from build123d import *

# Parameters (mm, degrees)
F1_DEPTH = 15
F3_DEPTH = 10


with BuildPart() as f1:
    # F0 (on Front) → F1 (new body)
    with BuildSketch(Plane.XZ):
        Polygon((-28.551763, 0), (-7.551763, 0), (-7.551763, 2), (-8.551763, 2), (-8.551763, 3), (-27.551763, 3), (-27.551763, 2), (-28.551763, 2), align=None)
    extrude(amount=F1_DEPTH)

    # F2 (on face) → F3 (cut)
    with BuildSketch(Plane(origin=(0, 0, 0), x_dir=(-1, 0, 0), z_dir=(0, 1, 0))):
        Polygon((8.051763, 1.5), (8.051763, 0.5), (9.301763, 0.5), (9.301763, 1), (9.801763, 1), (9.801763, 0.5), (10.301763, 0.5), (10.301763, 1), (10.801763, 1), (10.801763, 0.5), (11.301763, 0.5), (11.301763, 1), (11.801763, 1), (11.801763, 0.5), (12.301763, 0.5), (12.301763, 1), (12.801763, 1), (12.801763, 0.5), (13.301763, 0.5), (13.301763, 1), (13.801763, 1), (13.801763, 0.5), (14.301763, 0.5), (14.301763, 1), (14.801763, 1), (14.801763, 0.5), (15.301763, 0.5), (15.301763, 1), (15.801763, 1), (15.801763, 0.5), (16.301763, 0.5), (16.301763, 1), (16.801763, 1), (16.801763, 0.5), (17.301763, 0.5), (17.301763, 1), (17.801763, 1), (17.801763, 0.5), (18.301763, 0.5), (18.301763, 1), (18.801763, 1), (18.801763, 0.5), (19.301763, 0.5), (19.301763, 1), (19.801763, 1), (19.801763, 0.5), (20.301763, 0.5), (20.301763, 1), (20.801763, 1), (20.801763, 0.5), (21.301763, 0.5), (21.301763, 1), (21.801763, 1), (21.801763, 0.5), (22.301763, 0.5), (22.301763, 1), (22.801763, 1), (22.801763, 0.5), (23.301763, 0.5), (23.301763, 1), (23.801763, 1), (23.801763, 0.5), (24.301763, 0.5), (24.301763, 1), (24.801763, 1), (24.801763, 0.5), (25.301763, 0.5), (25.301763, 1), (25.801763, 1), (25.801763, 0.5), (26.301763, 0.5), (26.301763, 1), (26.831981, 1), (26.831981, 0.5), (28.081981, 0.5), (28.081981, 1.5), (27.081981, 1.5), (27.081981, 2.5), (26.301763, 2.5), (26.301763, 2), (25.801763, 2), (25.801763, 2.5), (25.301763, 2.5), (25.301763, 2), (24.801763, 2), (24.801763, 2.5), (24.301763, 2.5), (24.301763, 2), (23.801763, 2), (23.801763, 2.5), (23.301763, 2.5), (23.301763, 2), (22.801763, 2), (22.801763, 2.5), (22.301763, 2.5), (22.301763, 2), (21.801763, 2), (21.801763, 2.5), (21.301763, 2.5), (21.301763, 2), (20.801763, 2), (20.801763, 2.5), (20.301763, 2.5), (20.301763, 2), (19.801763, 2), (19.801763, 2.5), (19.301763, 2.5), (19.301763, 2), (18.801763, 2), (18.801763, 2.5), (18.301763, 2.5), (18.301763, 2), (17.801763, 2), (17.801763, 2.5), (17.301763, 2.5), (17.301763, 2), (16.801763, 2), (16.801763, 2.5), (16.301763, 2.5), (16.301763, 2), (15.801763, 2), (15.801763, 2.5), (15.301763, 2.5), (15.301763, 2), (14.801763, 2), (14.801763, 2.5), (14.301763, 2.5), (14.301763, 2), (13.801763, 2), (13.801763, 2.5), (13.301763, 2.5), (13.301763, 2), (12.801763, 2), (12.801763, 2.5), (12.301763, 2.5), (12.301763, 2), (11.801763, 2), (11.801763, 2.5), (11.301763, 2.5), (11.301763, 2), (10.801763, 2), (10.801763, 2.5), (10.301763, 2.5), (10.301763, 2), (9.801763, 2), (9.801763, 2.5), (9.051763, 2.5), (9.051763, 1.5), align=None)
    extrude(amount=-F3_DEPTH, mode=Mode.SUBTRACT)


solid = f1.part
Work out the finished part from the listing and answer in its coordinate system (mm). A direction names the side the tool comes from. Give positions to 0.01 mm unless a question says otherwise; leave off trailing zeros. Loops run counter-clockwise (first coordinate to the right, second up) from the corner with the lowest first, then second, coordinate; pieces in that order, holes last. Notation, with made-up numbers: (13.5, -25) - (69.5, -25) arc R10 cw to (69.5, -21) - close; hole circle Ø6 at (-30.5, 60.5). An arc over 180 degrees is marked (long way). Answer in a Markdown table with one row per item.
(1) Section A-A (z = 1.25) is taken. Give the vertices of the cut face in (x, y).
Results list:
| item | result |
|---|---|
| outline | (-28.55, -15) - (-7.55, -15) - (-7.55, 0) - (-8.05, 0) - (-8.05, -10) - (-28.08, -10) - (-28.08, 0) - (-28.55, 0) - close |
(2) Section B-B (y = -11.5) is taken. Give the vertices of the cut face in (x, z).
Results list:
| item | result |
|---|---|
| outline | (-28.55, 0) - (-7.55, 0) - (-7.55, 2) - (-8.55, 2) - (-8.55, 3) - (-27.55, 3) - (-27.55, 2) - (-28.55, 2) - close |
(3) Consider L1, parallel to Z at x = -20.25, y = -1; L2, parallel to Z at x = -12.5, y = -5.5; L3, parallel to X at y = -9.5, z = 1.9. Determine where each line is inside the solid, lowest interval first. Write a range as [from, to].
Results list:
| item | result |
|---|---|
| L1 | z = [0, 0.5], [2, 3] |
| L2 | z = [0, 1], [2.5, 3] |
| L3 | x = [-28.55, -27.08], [-9.05, -7.55] |
(4) A flat-ended cylindrical pin translates along its axis: pin 1 Ø0.6 at (x, y) = (-18, -7) entering from -Z. Find the tip coordinate at first contact, or state that the pin passes through.
Results list:
| item | result |
|---|---|
| pin 1 | stops at z = 0 |
(5) A tool of negligible diameter and unlimited length cuts with its end or side. For faces 1 (the face through (-27.552, -7.4, 2.5)), 2 (the face through (-8, -7, 2)), 3 (the face through (-27.082, -5, 2)), from which of +Z, -Z, +X, -X, +Y, -Y can it reach the whole face along a straight path? Write none if from no direction.
Results list:
| item | result |
|---|---|
| face 1 | +Z, -X, +Y, -Y |
| face 2 | +Z, +X, +Y, -Y |
| face 3 | +Y |
(6) For a pull along X with two mould halves and no side action, classify faces 4 (the face through (-28.082, -5, 1)), 5 (the face through (-18.2, 0, 0.2)), 6 (the face through (-8.552, -7.4, 2.5)), 7 (the face through (-27.6, -4.9, 1.5)) as pulls with the +X half, pulls with the -X half, needs draft (parallel to the pull), parting line crosses it, or undercut.
Results list:
| item | result |
|---|---|
| face 4 | undercut |
| face 5 | needs draft |
| face 6 | pulls with the +X half |
| face 7 | undercut |
